Verification items for the finished model (mm, model axes). A direction names the side the tool comes from. Round coordinates to 2 decimals unless told otherwise and drop trailing zeros. Order: outer loops, then holes, each group sorted by start corner. A loop starts at its lowest first (then second) coordinate and runs counter-clockwise, first axis right, second up. Notation, with made-up numbers: M -19,-31 L -3,-31 A23 ccw -3,2 Z; hole C -36,53 d8. An arc over 180 degrees is marked long. Use CSV: the item, a comma, the result in double quotes. Start each with the question number.
Q1. Sectioned sample at C-C (x = -5.5). Enter the section's corners in (y, z), and give its area (3 significant figures).
Q2. Scan lines: line 1 (X direction, y = -13, z = 5); line 2 (X direction, y = -20, z = 1.25); line 3 (Y direction, x = 36.5, z = 4.75). Record each from-to range of solid material in increasing order.
Q3. Sectioned sample at A-A (z = 5.5). Enter the section's corners in (x, y) (1 decimal), and give its area (3 significant figures).
Q4. Mould release check, pull along Y, two halves, no side actions. Record for faces 1 (the face through (-36, 33.25, 6.96)), 2 (the face through (-1, -49, 5)), 3 (the face through (40.56, 41.395, 4.93)): +Y half, -Y half, draft (parallel to the pull), parting line (faces both ways), or undercut.
Q5. Set-up check for faces 4 (the face through (32.4, 15.61, 2.03)), 5 (the face through (1, -40, 7)), 6 (the face through (-22, -41, 10)): record each of +Z, -Z, +X, -X, +Y, -Y from which the full face is reachable in a straight line by a thin tool's end or side.
Q6. Gauge pin test, flat ends, axial feed: pin 1 Ø1.6 at (x, z) = (-26.5, 1.5) entering from +Y; pin 2 Ø1.6 at (x, z) = (27.5, 2) entering from +Y; pin 3 Ø1.6 at (x, z) = (-45, 2.5) entering from +Y. Record the tip position at first contact, or that the pin passes through.
Q7. Sectioned sample at B-B (y = 17). Enter the section's corners in (x, z).
Q8. Sectioned sample at D-D (x = -23.5). State how many separate pieces and enclosed holes the cut face has, and give its area (3 significant figures).
```python
from build123d import *

# Parameters (mm, degrees)
F1_DEPTH = 4
F2_DEPTH = 10
F4_DEPTH = 25
F5_DEPTH = 5
F6_W     = 40
F6_H     = 2.5
F7_DEPTH = 25
F8_R     = 1


with BuildPart() as f1:
    # F0 (on Top) → F1 (new body)
    with BuildSketch(Plane.XY):
        Polygon((71, -40), (71, 26.6875), (0, 40), (-71, 26.6875), (-71, -40), align=None)
        Polygon((77, -46), (77, 25.5625), (74, 26.125), (74, -43), (-74, -43), (-74, 26.125), (-77, 25.5625), (-77, -46), align=None)
        Polygon((0, 43), (71, 29.6875), (71, 32.6875), (0, 46), (-71, 32.6875), (-71, 29.6875), align=None)
        Polygon((-80, -49), (80, -49), (80, 25), (77, 25.5625), (77, -46), (-77, -46), (-77, 25.5625), (-80, 25), align=None)
        Polygon((74, -43), (74, 26.125), (71, 26.6875), (71, -40), (-71, -40), (-71, 26.6875), (-74, 26.125), (-74, -43), align=None)
        Polygon((-80, 31), (-80, 28), (-77, 28.5625), (-77, 31.5625), align=None)
        Polygon((-80, 34), (-80, 31), (-77, 31.5625), (-77, 34.5625), align=None)
        Polygon((-80, 28), (-80, 25), (-77, 25.5625), (-77, 28.5625), align=None)
        Polygon((-77, 34.5625), (-77, 31.5625), (-74, 32.125), (-74, 35.125), align=None)
        Polygon((-77, 31.5625), (-77, 28.5625), (-74, 29.125), (-74, 32.125), align=None)
        Polygon((-77, 28.5625), (-77, 25.5625), (-74, 26.125), (-74, 29.125), align=None)
        Polygon((-74, 32.125), (-74, 29.125), (-71, 29.6875), (-71, 32.6875), align=None)
        Polygon((-74, 29.125), (-74, 26.125), (-71, 26.6875), (-71, 29.6875), align=None)
        Polygon((-74, 35.125), (-74, 32.125), (-71, 32.6875), (-71, 35.6875), align=None)
        Polygon((0, 46), (71, 32.6875), (71, 35.6875), (0, 49), (-71, 35.6875), (-71, 32.6875), align=None)
        Polygon((0, 40), (71, 26.6875), (71, 29.6875), (0, 43), (-71, 29.6875), (-71, 26.6875), align=None)
        Polygon((71, 32.6875), (74, 32.125), (74, 35.125), (71, 35.6875), align=None)
        Polygon((74, 32.125), (77, 31.5625), (77, 34.5625), (74, 35.125), align=None)
        Polygon((77, 31.5625), (80, 31), (80, 34), (77, 34.5625), align=None)
        Polygon((77, 28.5625), (80, 28), (80, 31), (77, 31.5625), align=None)
        Polygon((77, 25.5625), (80, 25), (80, 28), (77, 28.5625), align=None)
        Polygon((74, 26.125), (77, 25.5625), (77, 28.5625), (74, 29.125), align=None)
        Polygon((71, 26.6875), (74, 26.125), (74, 29.125), (71, 29.6875), align=None)
        Polygon((71, 29.6875), (74, 29.125), (74, 32.125), (71, 32.6875), align=None)
        Polygon((74, 29.125), (77, 28.5625), (77, 31.5625), (74, 32.125), align=None)
    extrude(amount=F1_DEPTH)

    # F0 (on Top) → F2 (join)
    with BuildSketch(Plane.XY):
        Polygon((77, 31.5625), (80, 31), (80, 34), (77, 34.5625), align=None)
        Polygon((74, 32.125), (77, 31.5625), (77, 34.5625), (74, 35.125), align=None)
        Polygon((71, 32.6875), (74, 32.125), (74, 35.125), (71, 35.6875), align=None)
        Polygon((0, 46), (71, 32.6875), (71, 35.6875), (0, 49), (-71, 35.6875), (-71, 32.6875), align=None)
        Polygon((-74, 35.125), (-74, 32.125), (-71, 32.6875), (-71, 35.6875), align=None)
        Polygon((-77, 34.5625), (-77, 31.5625), (-74, 32.125), (-74, 35.125), align=None)
        Polygon((-80, 34), (-80, 31), (-77, 31.5625), (-77, 34.5625), align=None)
        Polygon((-80, 28), (-80, 25), (-77, 25.5625), (-77, 28.5625), align=None)
        Polygon((-74, 29.125), (-74, 26.125), (-71, 26.6875), (-71, 29.6875), align=None)
        Polygon((0, 40), (71, 26.6875), (71, 29.6875), (0, 43), (-71, 29.6875), (-71, 26.6875), align=None)
        Polygon((77, 25.5625), (80, 25), (80, 28), (77, 28.5625), align=None)
        Polygon((71, 26.6875), (74, 26.125), (74, 29.125), (71, 29.6875), align=None)
        Polygon((-80, -49), (80, -49), (80, 25), (77, 25.5625), (77, -46), (-77, -46), (-77, 25.5625), (-80, 25), align=None)
        Polygon((74, -43), (74, 26.125), (71, 26.6875), (71, -40), (-71, -40), (-71, 26.6875), (-74, 26.125), (-74, -43), align=None)
        Polygon((-80, 31), (-80, 28), (-77, 28.5625), (-77, 31.5625), align=None)
        Polygon((77, 28.5625), (80, 28), (80, 31), (77, 31.5625), align=None)
    extrude(amount=F2_DEPTH)

    # F3 (on face) → F4 (cut)
    with BuildSketch(Plane.XY.offset(4)):
        with BuildLine():
            Line((-3.5, 0), (0, 0))
            Line((0, 0), (0, 3.5))
            ThreePointArc((0, 3.5), (-2.4748737342, 2.4748737342), (-3.5, 0))
        make_face()
        with BuildLine():
            Line((0, 3.5), (0, 0))
            Line((0, 0), (-3.5, 0))
            ThreePointArc((-3.5, 0), (0, -3.5), (3.5, 0))
            ThreePointArc((3.5, 0), (2.4748737342, 2.4748737342), (0, 3.5))
        make_face()
    extrude(amount=-F4_DEPTH, mode=Mode.SUBTRACT)

    # F3 (on face) → F5 (cut)
    with BuildSketch(Plane.XY.offset(4)):
        with BuildLine():
            ThreePointArc((-48.0253626304, 12.6815713362), (-50.7987183194, 8.6005751391), (-46.7353428851, 5.8014660276))
            Line((-46.7353428851, 5.8014660276), (-48.0253626304, 12.6815713362))
        make_face()
        Polygon((-46.7353428851, 5.8014660276), (-15.0502303624, 11.7424246256), (-16.3402501078, 18.6225299342), (-48.0253626304, 12.6815713362), align=None)
        with BuildLine():
            Line((-16.3402501078, 18.6225299342), (-15.0502303624, 11.7424246256))
            ThreePointArc((-15.0502303624, 11.7424246256), (-12.2805111805, 15.8227389776), (-16.3402501078, 18.6225299342))
        make_face()
        with BuildLine():
            ThreePointArc((16.3402501078, 18.6225299342), (12.2805111805, 15.8227389776), (15.0502303624, 11.7424246256))
            Line((15.0502303624, 11.7424246256), (46.7353428851, 5.8014660276))
            ThreePointArc((46.7353428851, 5.8014660276), (50.7987183194, 8.6005751391), (48.0253626304, 12.6815713362))
            Line((48.0253626304, 12.6815713362), (16.3402501078, 18.6225299342))
        make_face()
    extrude(amount=-F5_DEPTH, mode=Mode.SUBTRACT)

    # F6 (on face) → F7 (cut)
    with BuildSketch(Plane.XY.offset(4)):
        with Locations((-35, -30.25)):
            Rectangle(F6_W, F6_H)
        with Locations((-35, -19.75)):
            Rectangle(F6_W, F6_H)
        with Locations((35, -19.75)):
            Rectangle(F6_W, F6_H)
        with Locations((35, -30.25)):
            Rectangle(F6_W, F6_H)
        with Locations((-35, -9.25)):
            Rectangle(F6_W, F6_H)
        with Locations((35, -9.25)):
            Rectangle(F6_W, F6_H)
    extrude(amount=-F7_DEPTH, mode=Mode.SUBTRACT)

    # F8
    f8_edges = [f1.edges().sort_by_distance(p)[0] for p in [
        (-35, -31.5, 4),
        (-35, -29, 4),
        (-35, -21, 4),
        (-35, -18.5, 4),
        (-35, -10.5, 4),
        (-35, -8, 4),
        (-55, -9.25, 4),
        (-55, -19.75, 4),
        (-55, -30.25, 4),
        (-15, -30.25, 4),
        (-15, -19.75, 4),
        (-15, -9.25, 4),
        (15, -9.25, 4),
        (15, -19.75, 4),
        (15, -30.25, 4),
        (35, -29, 4),
        (35, -31.5, 4),
        (35, -18.5, 4),
        (15, -9.25, 0),
        (15, -19.75, 0),
        (35, -31.5, 0),
        (15, -30.25, 0),
        (35, -29, 0),
        (35, -21, 0),
        (35, -18.5, 0),
        (35, -8, 0),
        (35, -10.5, 0),
        (55, -30.25, 0),
        (55, -19.75, 0),
        (55, -9.25, 0),
        (-15, -30.25, 0),
        (-15, -19.75, 0),
        (-55, -30.25, 0),
        (-55, -19.75, 0),
        (-55, -9.25, 0),
        (-35, -21, 0),
        (-35, -29, 0),
        (-35, -31.5, 0),
        (-35, -10.5, 0),
        (-35, -8, 0),
        (-35, -18.5, 0),
        (-15, -9.25, 0),
        (55, -30.25, 4),
        (55, -19.75, 4),
        (35, -21, 4),
        (35, -10.5, 4),
        (35, -8, 4),
        (55, -9.25, 4),
    ]]
    fillet(f8_edges, radius=F8_R)


solid = f1.part
```
Verdict:
1,outline,"M -49,0 L 47.97,0 L 47.97,10 L 44.97,10 L 44.97,4 L 41.97,4 L 41.97,10 L 38.97,10 L 38.97,4 L -40,4 L -40,10 L -43,10 L -43,4 L -46,4 L -46,10 L -49,10 Z"
1,area,"460 mm²"
2,line 1,"x = -80 to -77, -74 to -71, 71 to 74, 77 to 80"
2,line 2,"x = -80 to -55, -15 to 15, 55 to 80"
2,line 3,"y = -49 to -46, -43 to -40, 33.16 to 36.16, 39.16 to 42.16"
3,outline,"M -80,-49 L 80,-49 L 80,34 L 0,49 L -80,34 Z; M -74,-43 L 74,-43 L 74,29.1 L 0,43 L -74,29.1 Z; hole M -77,-46 L 77,-46 L 77,31.6 L 0,46 L -77,31.6 Z; hole M -71,-40 L 71,-40 L 71,26.7 L 0,40 L -71,26.7 Z"
3,area,"2,710 mm²"
4,face 1,"undercut"
4,face 2,"-Y half"
4,face 3,"+Y half"
5,face 4,"+Z, -Z"
5,face 5,"+Z"
5,face 6,"+Z, +X, -X, +Y, -Y"
6,pin 1,"stops at y = 44.18"
6,pin 2,"stops at y = 43.99"
6,pin 3,"stops at y = 40.71"
7,outline,"M -80,0 L -24.99,0 L -24.99,4 L -71,4 L -71,10 L -74,10 L -74,4 L -77,4 L -77,10 L -80,10 Z; M -12.73,0 L 12.73,0 L 12.73,4 L -12.73,4 Z; M 24.99,0 L 80,0 L 80,10 L 77,10 L 77,4 L 74,4 L 74,10 L 71,10 L 71,4 L 24.99,4 Z"
8,separate pieces,"5"
8,enclosed holes,"0"
8,area,"385 mm²"
